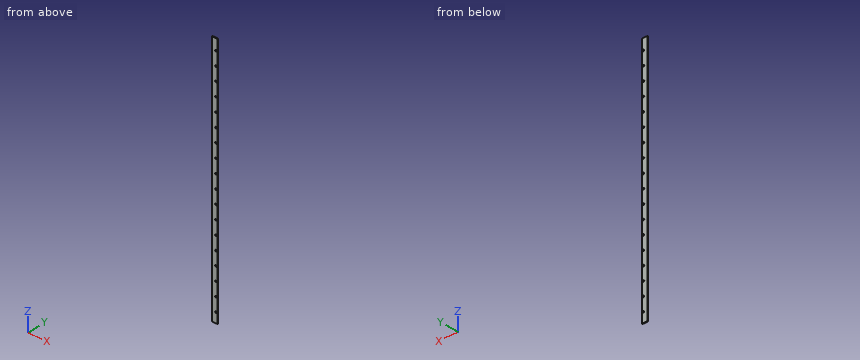
```python
from build123d import *

# Parameters (mm, degrees)
F0_W     = 39.5
F0_H     = 1855
F0_R     = 5.5
F1_DEPTH = 5


with BuildPart() as f1:
    # F0 (on Front) → F1 (new body)
    with BuildSketch(Plane.XZ):
        with Locations((-183.987974, 903.800355)):
            Rectangle(F0_W, F0_H)
        with Locations((-175.237974, 49.300355)):
            Circle(F0_R, mode=Mode.SUBTRACT)
        with Locations((-175.237974, 149.300355)):
            Circle(F0_R, mode=Mode.SUBTRACT)
        with Locations((-175.237974, 249.300355)):
            Circle(F0_R, mode=Mode.SUBTRACT)
        with Locations((-175.237974, 349.300355)):
            Circle(F0_R, mode=Mode.SUBTRACT)
        with Locations((-175.237974, 449.300355)):
            Circle(F0_R, mode=Mode.SUBTRACT)
        with Locations((-175.237974, 549.300355)):
            Circle(F0_R, mode=Mode.SUBTRACT)
        with Locations((-175.237974, 649.300355)):
            Circle(F0_R, mode=Mode.SUBTRACT)
        with Locations((-175.237974, 749.300355)):
            Circle(F0_R, mode=Mode.SUBTRACT)
        with Locations((-175.237974, 849.300355)):
            Circle(F0_R, mode=Mode.SUBTRACT)
        with Locations((-175.237974, 949.300355)):
            Circle(F0_R, mode=Mode.SUBTRACT)
        with Locations((-175.237974, 1049.300355)):
            Circle(F0_R, mode=Mode.SUBTRACT)
        with Locations((-175.237974, 1149.300355)):
            Circle(F0_R, mode=Mode.SUBTRACT)
        with Locations((-175.237974, 1249.300355)):
            Circle(F0_R, mode=Mode.SUBTRACT)
        with Locations((-175.237974, 1349.300355)):
            Circle(F0_R, mode=Mode.SUBTRACT)
        with Locations((-175.237974, 1449.300355)):
            Circle(F0_R, mode=Mode.SUBTRACT)
        with Locations((-175.237974, 1549.300355)):
            Circle(F0_R, mode=Mode.SUBTRACT)
        with Locations((-175.237974, 1649.300355)):
            Circle(F0_R, mode=Mode.SUBTRACT)
        with Locations((-175.237974, 1749.300355)):
            Circle(F0_R, mode=Mode.SUBTRACT)
    extrude(amount=F1_DEPTH)


solid = f1.part
```
The model under review builds one solid part; all positions refer to its coordinate system, in mm. Coordinates: 2 decimals unless noted, no trailing zeros. Answer in a Markdown table with one row per item. Add a question column.
Item 1: Clearance check with flat-ended pins moving along their axes: pin 1 (6.5 mm diameter, centred on x = -175.24, z = 949.3, fed in from -Y); pin 2 (17.5 mm diameter, centred on x = -175.24, z = 1649.3, fed in from -Y). State where each tip first meets the part, or that it passes through.
Item 2: We need section A-A on y = -1.4. Give the number of separate pieces and of enclosed holes in the cut face, plus the area to 3 significant figures.
Item 3: To check wall thickness, follow probe 1 along X at (y, z) = (-1.25, 1546.5); probe 2 along X at (y, z) = (-3.9, 844.5). State the ranges of each line that lie inside material, in increasing order.
Final values:
| question | item | result |
|---|---|---|
| 1 | pin 1 | passes through |
| 1 | pin 2 | stops at y = -5 |
| 2 | separate pieces | 1 |
| 2 | enclosed holes | 18 |
| 2 | area | 71,600 mm2 |
| 3 | probe 1 | x = -203.74 to -179.97, -170.5 to -164.24 |
| 3 | probe 2 | x = -203.74 to -177.92, -172.55 to -164.24 |
